Read the model definition and answer for the solid it produces. Units are mm, in the model's axes. Face numbers are marked on the shaded views. A direction names the side the tool comes from. Give positions to 0.01 mm unless a question says otherwise; leave off trailing zeros. Write each loop counter-clockwise with the first axis right and the second up, starting at its lowest first coordinate (ties: lowest second). Pieces come first, ordered by that corner, then holes. Notation, with made-up numbers: (67, 8) - (107, 8) arc R15 cw to (107, 15) - close; hole circle Ø6 at (4.25, -39). An arc over 180 degrees is marked (long way). Answer as a JSON object with one key per item and string values. Group by question number.
```python
from build123d import *

# Parameters (mm, degrees)
F0_W     = 40
F0_H     = 3
F0_W_2   = 3
F1_DEPTH = 40
F4_DEPTH = 40.001


with BuildPart() as f1:
    # F0 (on Top) → F1 (new body)
    with BuildSketch(Plane.XY):
        with Locations((-20, 1.5)):
            Rectangle(F0_W, F0_H)
        Polygon((0, 3), (0, 0), (9, 0), (9, 3), (6, 3), align=None)
        Polygon((-40, 3), (0, 3), (-40, 43), align=None)
        with Locations((7.5, 4.5)):
            Rectangle(F0_W_2, F0_H)
    extrude(amount=F1_DEPTH)

    # F3 (on face) → F4 (cut, through all)
    with BuildSketch(Plane.XY.offset(40)):
        Polygon((-4.242641, 3), (-37, 35.757359), (-37, 3), align=None)
    extrude(amount=-F4_DEPTH, mode=Mode.SUBTRACT)


solid = f1.part
```
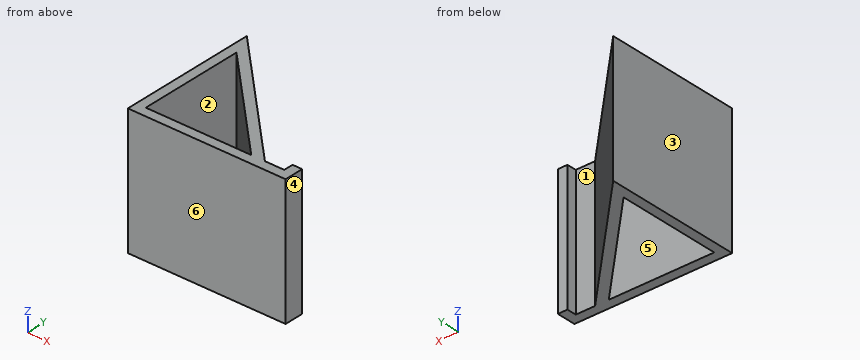
1) For a pull along Y with two mould halves and no side action, classify the marked faces 4, 5 and 6 as released by +Y, released by -Y, zero draft, split by the parting line, or undercut.
2) Find section C-C, the plane x = -34. Write down the section's boundary in (y, z), and give its area (3 significant figures).
3) Find section D-D, the plane x = -2.5. Write down the section's boundary in (y, z), and give its area (3 significant figures).
4) Find section B-B, the plane y = 22.5. Write down the section's boundary in (x, z), and give its area (3 significant figures).
5) Flat-ended cylindrical pins translate along their axes: pin 1 Ø12 at (x, z) = (-11.5, 14) entering from +Y; pin 2 Ø10 at (y, z) = (29, 8.5) entering from +X; pin 3 Ø6.5 at (x, z) = (4, 23) entering from +Y. Find the tip coordinate at first contact, or state that the pin passes through.
6) Which of the six approach directions +Z, -Z, +X, -X, +Y, -Y give full straight-line access (tool end or side, diameter ignored) to the marked faces 1, 2 and 3?
7) Find section A-A, the plane z = 8. Write down the section's boundary in (x, y).
8) Find the intervals of material crossed by line 1 (Y direction, x = 3, z = 26); line 2 (Y direction, x = -25.5, z = 15); line 3 (Y direction, x = -3, z = 7.5), in increasing order. Write a range as [from, to].
Values follow:
{
 "1": {"face 4": "zero draft", "face 5": "undercut", "face 6": "released by -Y"},
 "2": {"outline": "(0, 0) - (3, 0) - (3, 40) - (0, 40) - close; (32.76, 0) - (37, 0) - (37, 40) - (32.76, 40) - close", "area": "290 mm2"},
 "3": {"outline": "(0, 0) - (5.5, 0) - (5.5, 40) - (0, 40) - close", "area": "220 mm2"},
 "4": {"outline": "(-40, 0) - (-37, 0) - (-37, 40) - (-40, 40) - close; (-23.74, 0) - (-19.5, 0) - (-19.5, 40) - (-23.74, 40) - close", "area": "290 mm2"},
 "5": {"pin 1": "stops at y = 20.5", "pin 2": "stops at x = -21", "pin 3": "stops at y = 6"},
 "6": {"face 1": "+Z, -Z, +Y", "face 2": "+Z, -Z", "face 3": "+Z, -Z, -X, +Y, -Y"},
 "7": {"outline": "(-40, 0) - (9, 0) - (9, 6) - (6, 6) - (6, 3) - (0, 3) - (-40, 43) - close; hole (-37, 3) - (-4.24, 3) - (-37, 35.76) - close"},
 "8": {"line 1": "y = [0, 3]", "line 2": "y = [0, 3], [24.26, 28.5]", "line 3": "y = [0, 6]"}
}
